```python
from build123d import *

# Parameters (mm, degrees)
F0_R     = 6.35
F1_DEPTH = 1.6002
F2_R     = 4.7625
F3_DEPTH = 4.7498
F4_R     = 3.175
F5_DEPTH = 12.7


with BuildPart() as f1:
    # F0 (on Front) → F1 (new body)
    with BuildSketch(Plane.XZ):
        Circle(F0_R)
    extrude(amount=-F1_DEPTH)

    # F2 (on face) → F3 (join)
    with BuildSketch(Plane.XZ):
        Circle(F2_R)
    extrude(amount=F3_DEPTH)

    # F4 (on face) → F5 (cut, symmetric)
    with BuildSketch(Plane.XZ):
        Circle(F4_R)
    extrude(amount=F5_DEPTH, both=True, mode=Mode.SUBTRACT)


solid = f1.part
```
The listing builds one solid part. Answer for the finished solid, in the listing's coordinates (mm). A direction names the side the tool comes from. Coordinates: 2 decimals unless noted, no trailing zeros. Loops run counter-clockwise (first coordinate to the right, second up) from the corner with the lowest first, then second, coordinate; pieces in that order, holes last. Notation, with made-up numbers: (70, 48.5) - (94, 48.5) arc R13 cw to (94, 66.5) - close; hole circle Ø9 at (84.5, 88.5). An arc over 180 degrees is marked (long way). Write item = value, one per line.
1) Which of the six approach directions +Z, -Z, +X, -X, +Y, -Y give full straight-line access (tool end or side, diameter ignored) to faces 4 (the face through (-2, 1.6, 3)), 5 (the face through (-3.78, -2.34, -2.9))?
Responses:
face_4 = +Z, -Z, +X, -X, +Y
face_5 = -Y
2) Find the intervals of material crossed by line 1 along Z through (x, y) = (0, -1.5) (1 decimal); line 2 along Z through (x, y) = (0, 0.25) (3 decimals); line 3 along X through (y, z) = (-3, 1.5), in increasing order.
Responses:
line_1 = -4.8 to -3.2, 3.2 to 4.8
line_2 = -6.35 to -3.175, 3.175 to 6.35
line_3 = -4.52 to -2.8, 2.8 to 4.52
3) Section D-D (z = -3.75) is taken. Determine the outline of the cut face in (x, y).
Responses:
outline = (-5.12, 0) - (-2.94, 0) - (-2.94, -4.75) - (2.94, -4.75) - (2.94, 0) - (5.12, 0) - (5.12, 1.6) - (-5.12, 1.6) - close
4) Determine the mould class of faces 1 (the face through (1, 0, 5)), 2 (the face through (-0.69, -1.62, -3.1)), 3 (the face through (-1.38, 0.79, -6.2)) for opening direction Z: pulls with the +Z half, pulls with the -Z half, needs draft (parallel to the pull), parting line crosses it, or undercut.
Responses:
face_1 = needs draft
face_2 = undercut
face_3 = parting line crosses it
5) Each of these flat-tipped pins is pushed along its axis until it touches: P1, Ø3, axis at x = 5, z = -2, coming from the -Y side; P2, Ø5.5, axis at x = 0, z = 0, coming from the -Y side; P3, Ø1.5, axis at x = 4.5, y = -1.5, coming from the -Z side. Where does it stop, or does it pass through?
Responses:
P1 = -4.75
P2 = through
P3 = -2.94
